```python
from build123d import *

# Parameters (mm, degrees)
SKETCH_1_R      = 11
EXTRUDE_1_DEPTH = 21.5


with BuildPart() as part:
    # Эскиз1 → Бобышка-Вытянуть1 (new, symmetric)
    with BuildSketch(Plane(origin=(0, 0, 0), x_dir=(1, 0, 0), z_dir=(0, 1, 0))):
        with BuildLine():
            ThreePointArc((0, 13.5), (-9.545941546, 17.454058454), (-13.5, 27))
            Line((-13.5, 27), (-13.5, 30))
            Line((-13.5, 30), (-73.5, 30))
            Line((-73.5, 30), (-73.5, -30))
            Line((-73.5, -30), (-13.5, -30))
            Line((-13.5, -30), (-13.5, -27))
            ThreePointArc((-13.5, -27), (-9.545941546, -17.454058454), (0, -13.5))
            ThreePointArc((0, -13.5), (9.545941546, -9.545941546), (13.5, 0))
            ThreePointArc((13.5, 0), (9.545941546, 9.545941546), (0, 13.5))
        make_face()
        with Locations(Location((0, 0, 0), (0, 0, 270))):
            Circle(SKETCH_1_R, mode=Mode.SUBTRACT)
    extrude(amount=EXTRUDE_1_DEPTH, both=True)


solid = part.part
```
Can you work these out from the model? Positions are in its coordinate system, mm. A direction names the side the tool comes from. Give positions to 0.01 mm unless a question says otherwise; leave off trailing zeros. Loops run counter-clockwise (first coordinate to the right, second up) from the corner with the lowest first, then second, coordinate; pieces in that order, holes last. Notation, with made-up numbers: M 17.5,11.5 L 66.5,11.5 A17 cw 66.5,23.5 Z; hole C 1.5,85 d1. An arc over 180 degrees is marked long. Use one line per item in the form item = value. Start each with the question number.
(1) I want a section at D-D, the plane z = -25.5. Write out the boundary of the cut face in (x, y).
(2) Please list where these lines run through material, in increasing order: line 1 (X direction, y = -6.5, z = 0); line 2 (Z direction, x = 2, y = 1); line 3 (X direction, y = -7, z = 10).
(3) I want a section at C-C, the plane x = -7. Write out the boundary of the cut face in (y, z), and give its area (3 significant figures).
(4) I want a section at B-B, the plane z = 4.5. Write out the boundary of the cut face in (x, y), and give its area (3 significant figures).
(5) I want a section at A-A, the plane y = 4.5. Write out the boundary of the cut face in (x, z).
(6) On a 3-axis mill with a long thin cutter (end or side, diameter ignored), from which of +Z, -Z, +X, -X, +Y, -Y can I reach the whole of each face in a straight line? I mean faces 1 (the flat face through (-13.5, 0, -28)), 2 (the flat face through (-44, 0, 30)), 3 (the flat face through (-13.5, 0, 29)). Say none if no direction works.
(7) I'm going to push flat-ended pins straight in: P1, Ø3.5, axis at y = -2, z = 28.5, coming from the +X side; P2, Ø6, axis at y = -16.5, z = -7.5, coming from the +X side. Where does each tip first touch, or does it pass through?
Worked out:
q1.outline = M -73.5,-21.5 L -13.42,-21.5 L -13.42,21.5 L -73.5,21.5 Z
q2.line_1 = -73.5 to -11, 11 to 13.5
q2.line_2 = -13.35 to -10.82, 10.82 to 13.35
q2.line_3 = -73.5 to -4.58, 4.58 to 9.07
q3.outline = M -21.5,-15.46 L 21.5,-15.46 L 21.5,-8.49 L -21.5,-8.49 Z; M -21.5,8.49 L 21.5,8.49 L 21.5,15.46 L -21.5,15.46 Z
q3.area = 600 mm²
q4.outline = M -73.5,-21.5 L -10.04,-21.5 L -10.04,21.5 L -73.5,21.5 Z; M 10.04,-21.5 L 12.73,-21.5 L 12.73,21.5 L 10.04,21.5 Z
q4.area = 2,840 mm²
q5.outline = M -73.5,-30 L -13.5,-30 L -13.5,-27 A13.5 cw 0,-13.5 A13.5 ccw 0,13.5 A13.5 cw -13.5,27 L -13.5,30 L -73.5,30 Z; hole C 0,0 d22
q6.face_1 = -Z, +X, +Y, -Y
q6.face_2 = +Z, +X, -X, +Y, -Y
q6.face_3 = +Z, +X, +Y, -Y
q7.P1 = -13.5
q7.P2 = 12.73
